```python
from build123d import *

# Parameters (mm, degrees)
BOSS_EXTRUDE1_DEPTH         = 6.35
SKETCH3_W                   = 165.1
SKETCH3_H                   = 184.15
CUT_EXTRUDE1_DEPTH          = 7.35
F_1_4_CLEARANCE_HOLE1_D     = 5.1054
F_1_4_CLEARANCE_HOLE1_DEPTH = 25.4
F_1_4_CLEARANCE_HOLE1_TIP   = 1.533816902


with BuildPart() as part:
    # Sketch1 → Boss-Extrude1 (new body)
    with BuildSketch(Plane(origin=(0, 0, 0), x_dir=(0, 0, -1), z_dir=(1, 0, 0))):
        Polygon((257.81, 0), (-257.81, 0), (-95.25, 227.241295543), (95.25, 227.241295543), align=None)
    extrude(amount=BOSS_EXTRUDE1_DEPTH)

    # Sketch3 → Cut-Extrude1 (cut, through all)
    with BuildSketch(Plane(origin=(6.35, 0, 0), x_dir=(0, 0, -1), z_dir=(1, 0, 0))):
        with Locations((0, 118.656295543)):
            Rectangle(SKETCH3_W, SKETCH3_H)
    extrude(amount=-CUT_EXTRUDE1_DEPTH, mode=Mode.SUBTRACT)

    # 1/4 Clearance Hole1
    with Locations(Plane.ZY):
        with Locations((19.05, 217.081295543), (-50.8, 217.081295543), (-50.8, 151.464628876), (-50.8, 85.84796221), (-50.8, 20.231295543), (19.05, 20.231295543), (88.9, 20.231295543), (88.9, 85.84796221), (88.9, 151.464628876), (88.9, 217.081295543)):
            Hole(F_1_4_CLEARANCE_HOLE1_D / 2, depth=F_1_4_CLEARANCE_HOLE1_DEPTH)
            with Locations((0, 0, -(F_1_4_CLEARANCE_HOLE1_DEPTH + F_1_4_CLEARANCE_HOLE1_TIP / 2))):  # 118° drill point
                Cone(0, F_1_4_CLEARANCE_HOLE1_D / 2, F_1_4_CLEARANCE_HOLE1_TIP, mode=Mode.SUBTRACT)


solid = part.part
```
Build history of the part. All positions in model axes, mm. Coordinates: 2 decimals unless noted, no trailing zeros. Write each loop counter-clockwise with the first axis right and the second up, starting at its lowest first coordinate (ties: lowest second). Pieces come first, ordered by that corner, then holes.
1. Drop flat-ended pins along their axis: pin 1 (4.5 mm diameter, centred on y = 20.23, z = 88.9, fed in from +X); pin 2 (1 mm diameter, centred on x = 4, y = 170.5, fed in from +Z); pin 3 (1.5 mm diameter, centred on x = 4.5, y = 58, fed in from -Z); pin 4 (1 mm diameter, centred on x = 4, y = 183, fed in from -Z). Give the stop position or say it passes through.
Answer block:
pin 1: passes through
pin 2: stops at z = 136.2
pin 3: stops at z = -216.86
pin 4: stops at z = -127.26
2. Band-saw the part on C-C, the plane x = 1.75. Give the number of separate pieces and of enclosed holes in the cut face, and give its area (3 significant figures).
Answer block:
separate pieces: 1
enclosed holes: 9
area: 49,700 mm2
3. Drill centre lines: probe 1 along Y at (x, z) = (2.75, 88.9); probe 2 along Y at (x, z) = (3.25, -50.8); probe 3 along Y at (x, z) = (3.75, -49). Where is each one in solid material? Low to high.
Answer block:
probe 1: y = 0 to 17.68, 22.78 to 83.3, 88.4 to 148.91, 154.02 to 214.53, 219.63 to 227.24
probe 2: y = 0 to 17.68, 22.78 to 26.58, 210.73 to 214.53, 219.63 to 227.24
probe 3: y = 0 to 18.42, 22.04 to 26.58, 210.73 to 215.27, 218.89 to 227.24
4. Band-saw the part on B-B, the plane y = 113. Give the cut face in (x, z), and give its area (3 significant figures).
Answer block:
outline: (0, -176.97) - (6.35, -176.97) - (6.35, -82.55) - (0, -82.55) - close; (0, 82.55) - (6.35, 82.55) - (6.35, 176.97) - (0, 176.97) - close
area: 1,200 mm2
5. Band-saw the part on A-A, the plane z = 43. Give the cut face in (x, y), and give its area (3 significant figures).
Answer block:
outline: (0, 0) - (6.35, 0) - (6.35, 26.58) - (0, 26.58) - close; (0, 210.73) - (6.35, 210.73) - (6.35, 227.24) - (0, 227.24) - close
area: 274 mm2
